Work out the finished part from the listing and answer in its coordinate system (mm). Face numbers are marked on the shaded views. A direction names the side the tool comes from. Give positions to 0.01 mm unless a question says otherwise; leave off trailing zeros. Loops run counter-clockwise (first coordinate to the right, second up) from the corner with the lowest first, then second, coordinate; pieces in that order, holes last. Notation, with made-up numbers: (-9.75, 21.25) -> (5.25, 21.25) arc R8 cw to (5.25, 28.25) -> close; hole circle Ø6 at (62.5, -7). An arc over 180 degrees is marked (long way). Answer as CSV lines item,"result". Start each with the question number.
1. Flat-ended cylindrical pins translate along their axes: pin 1 Ø1 at (y, z) = (37.5, -2) entering from -X; pin 2 Ø5 at (x, z) = (44.5, -11.5) entering from -Y (3 decimals); pin 3 Ø5 at (y, z) = (28, 33) entering from -X. Find the tip coordinate at first contact, or state that the pin passes through.
2. Find section B-B, the plane x = 15.5. Count the separate pieces of the cut face and the enclosed holes in it, and give its area (3 significant figures).
3. Find section A-A, the plane z = 39. Give the vertices of the cut face in (x, y) (1 decimal).
4. Find the intervals of material crossed by line 1 along Z through (x, y) = (17, 15); line 2 along X through (y, z) = (15, 35.5) (1 decimal); line 3 along Y through (x, z) = (16, -29), in increasing order.
5. Determine the mould class of the marked faces 1, 2, 3 and 4 for opening direction Z: +Z half, -Z half, draft (parallel to the pull), parting line (faces both ways), or undercut.
6. A tool of negligible diameter and unlimited length cuts with its end or side. For the marked faces 5, 6, 7 and 8, from which of +Z, -Z, +X, -X, +Y, -Y can it reach the whole face along a straight path? Write none if from no direction.
from build123d import *

# Parameters (mm, degrees)
BOSS_EXTRUDE1_DEPTH = 51.59375
BOSS_EXTRUDE2_DEPTH = 75.156571292
SKETCH5_R           = 7.9375
CUT_EXTRUDE1_DEPTH  = 109.930311747
SKETCH6_R           = 6.35
CUT_EXTRUDE2_DEPTH  = 76.68979598


with BuildPart() as part:
    # Sketch2 → Boss-Extrude1 (new, symmetric)
    with BuildSketch(Plane.XY):
        Polygon((0, 9.525), (-15.875, 9.525), (-15.875, 25.4), (49.2125, 25.4), (49.2125, 9.525), (33.3375, 9.525), (33.3375, 0), (0, 0), align=None)
    extrude(amount=BOSS_EXTRUDE1_DEPTH, both=True)

    # Sketch3 → Boss-Extrude2 (add, along a direction that is not the sketch's normal)
    with BuildSketch(Plane(origin=(49.2125, 0, 0), x_dir=(0, 0, -1), z_dir=(1, 0, 0))):
        with BuildLine():
            Line((0.79375, 25.4), (-37.30625, 25.4))
            ThreePointArc((-37.30625, 25.4), (-18.25625, 44.45), (0.79375, 25.4))
        make_face()
    extrude(amount=-BOSS_EXTRUDE2_DEPTH, dir=(0.86602540378444, 0, 0.49999999999999767))

    # Sketch5 → Cut-Extrude1 (cut, through all, along a direction that is not the sketch's normal)
    with BuildSketch(Plane(origin=(49.2125, 0, 0), x_dir=(0, 0, -1), z_dir=(1, 0, 0))):
        with Locations((-18.25625, 25.4)):
            Circle(SKETCH5_R)
    extrude(amount=-CUT_EXTRUDE1_DEPTH, dir=(0.86602540378444, 0, 0.49999999999999767), mode=Mode.SUBTRACT)

    # Sketch6 → Cut-Extrude2 (cut, through all)
    with BuildSketch(Plane(origin=(0, 25.4, 0), x_dir=(1, 0, 0), z_dir=(0, 1, 0))):
        with Locations(Location((16.66875, -37.30625, 0), (0, 0, 180))):
            Circle(SKETCH6_R)
        with Locations(Location((16.66875, 37.30625, 0), (0, 0, 180))):
            Circle(SKETCH6_R)
    extrude(amount=-CUT_EXTRUDE2_DEPTH, mode=Mode.SUBTRACT)


solid = part.part
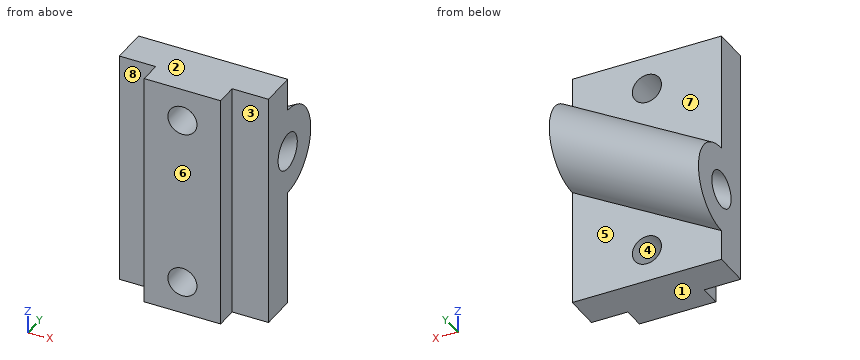
Resolved:
1,pin 1,"stops at x = -12.47"
1,pin 2,"stops at y = 9.525"
1,pin 3,"stops at x = 37.7"
2,separate pieces,"3"
2,enclosed holes,"1"
2,area,"2,360 mm^2"
3,outline,"(-15.9, 9.5) -> (0, 9.5) -> (0, 0) -> (10.5, 0) -> (10.5, 25.4) -> (-15.9, 25.4) -> close; (22.8, 0) -> (33.3, 0) -> (33.3, 9.5) -> (49.2, 9.5) -> (49.2, 25.4) -> (22.8, 25.4) -> close"
4,line 1,"z = -51.59 to -43.65, -30.96 to 30.96, 43.65 to 51.59"
4,line 2,"x = -15.9 to 10.6, 22.8 to 49.2"
4,line 3,"y = 0 to 25.4"
5,face 1,"-Z half"
5,face 2,"+Z half"
5,face 3,"draft"
5,face 4,"undercut"
6,face 5,"-Z, +X, +Y"
6,face 6,"+Z, -Z, +X, -X, -Y"
6,face 7,"+Z, -X, +Y"
6,face 8,"+Z, -Z, -X, -Y"
